Could you check a few things on this model? Use its own coordinates, in mm. A direction names the side the tool comes from. Round coordinates to 2 decimals unless told otherwise and drop trailing zeros. Loops run counter-clockwise (first coordinate to the right, second up) from the corner with the lowest first, then second, coordinate; pieces in that order, holes last.
from build123d import *

# Parameters (mm, degrees)
SKETCH_1_R      = 1.5
EXTRUDE_1_DEPTH = 2.2
FILLET_1_R      = 1


with BuildPart() as part:
    # 草图1 → 凸台-拉伸1 (new body)
    with BuildSketch(Plane(origin=(0, 0, 0), x_dir=(0, 0, -1), z_dir=(1, 0, 0))):
        Polygon((-14.5, -10), (23.5, -10), (23.5, 10), (-14.5, 10), (-14.5, 12), (-21.5, 12), (-21.5, 10), (-23.5, 10), (-23.5, -10), (-21.5, -10), (-21.5, -12), (-14.5, -12), align=None)
        with BuildLine():
            ThreePointArc((-15.845, -6.995), (-16.139357685, -7.705642315), (-16.85, -8))
            Line((-16.85, -8), (-19.15, -8))
            ThreePointArc((-19.15, -8), (-20.155, -6.995), (-19.15, -5.99))
            Line((-19.15, -5.99), (-19.15, 5.99))
            ThreePointArc((-19.15, 5.99), (-20.155, 6.995), (-19.15, 8))
            Line((-19.15, 8), (-16.85, 8))
            ThreePointArc((-16.85, 8), (-16.139357685, 7.705642315), (-15.845, 6.995))
            ThreePointArc((-15.845, 6.995), (-16.139357685, 6.284357685), (-16.85, 5.99))
            Line((-16.85, 5.99), (-16.85, -5.99))
            ThreePointArc((-16.85, -5.99), (-16.139357685, -6.284357685), (-15.845, -6.995))
        make_face(mode=Mode.SUBTRACT)
        with BuildLine():
            Line((10, -7), (-10.85, -7))
            ThreePointArc((-10.85, -7), (-12.275, -5.575), (-10.85, -4.15))
            Line((-10.85, -4.15), (10, -4.15))
            ThreePointArc((10, -4.15), (11.425, -5.575), (10, -7))
        make_face(mode=Mode.SUBTRACT)
        with BuildLine():
            Line((-3.01, -1.15), (-8.99, -1.15))
            ThreePointArc((-8.99, -1.15), (-9.995, -2.155), (-11, -1.15))
            Line((-11, -1.15), (-11, 1.15))
            ThreePointArc((-11, 1.15), (-9.995, 2.155), (-8.99, 1.15))
            Line((-8.99, 1.15), (-3.01, 1.15))
            ThreePointArc((-3.01, 1.15), (-2.005, 2.155), (-1, 1.15))
            Line((-1, 1.15), (-1, -1.15))
            ThreePointArc((-1, -1.15), (-2.005, -2.155), (-3.01, -1.15))
        make_face(mode=Mode.SUBTRACT)
        with Locations((16, -5)):
            Circle(SKETCH_1_R, mode=Mode.SUBTRACT)
        with BuildLine():
            ThreePointArc((-10.85, 4.15), (-12.275, 5.575), (-10.85, 7))
            Line((-10.85, 7), (10, 7))
            ThreePointArc((10, 7), (11.425, 5.575), (10, 4.15))
            Line((10, 4.15), (-10.85, 4.15))
        make_face(mode=Mode.SUBTRACT)
        with BuildLine():
            Line((16.99, -1.15), (11.01, -1.15))
            ThreePointArc((11.01, -1.15), (10.005, -2.155), (9, -1.15))
            Line((9, -1.15), (9, 1.15))
            ThreePointArc((9, 1.15), (10.005, 2.155), (11.01, 1.15))
            Line((11.01, 1.15), (16.99, 1.15))
            ThreePointArc((16.99, 1.15), (17.995, 2.155), (19, 1.15))
            Line((19, 1.15), (19, -1.15))
            ThreePointArc((19, -1.15), (17.995, -2.155), (16.99, -1.15))
        make_face(mode=Mode.SUBTRACT)
        with Locations((16, 5)):
            Circle(SKETCH_1_R, mode=Mode.SUBTRACT)
    extrude(amount=EXTRUDE_1_DEPTH)

    # 圆角1
    fillet_1_edges = [part.edges().sort_by_distance(p)[0] for p in [
        (1.1, -10, 23.5),
        (1.1, 10, 23.5),
        (1.1, 12, 14.5),
        (1.1, 10, 14.5),
        (1.1, 10, -23.5),
        (1.1, -10, -23.5),
        (1.1, -10, 14.5),
        (1.1, -12, 14.5),
        (1.1, -12, 21.5),
        (1.1, -10, 21.5),
        (1.1, 12, 21.5),
        (1.1, 10, 21.5),
    ]]
    fillet(fillet_1_edges, radius=FILLET_1_R - 0.0001)  # a hair under: the kernel refuses the full size


solid = part.part
Item 1: Will these pins go through, and if not, where does the flat tip stop? pin 1 (1.1 mm diameter, centred on x = 1.5, z = 5.5, fed in from -Y); pin 2 (3 mm diameter, centred on y = 3, z = 15.5, fed in from -X); pin 3 (0.7 mm diameter, centred on x = 0.5, z = 5, fed in from +Y).
Results list:
pin 1: stops at y = -10
pin 2: stops at x = 0
pin 3: stops at y = 10
Item 2: If we section it at A-A, the plane z = -8: Please give me the cut outline in (x, y), then the cut area to 3 significant figures.
Results list:
outline: (0, -10) - (2.2, -10) - (2.2, -7) - (0, -7) - close; (0, -4.15) - (2.2, -4.15) - (2.2, 4.15) - (0, 4.15) - close; (0, 7) - (2.2, 7) - (2.2, 10) - (0, 10) - close
area: 31.5 mm2
Item 3: If we section it at D-D, the plane y = -7.5: Please give me the cut outline in (x, z), then the cut area to 3 significant figures.
Results list:
outline: (0, -23.5) - (2.2, -23.5) - (2.2, 15.98) - (0, 15.98) - close; (0, 20.02) - (2.2, 20.02) - (2.2, 23.5) - (0, 23.5) - close
area: 94.5 mm2
Item 4: If we section it at B-B, the plane y = 5: Please give me the cut outline in (x, z), then the cut area to 3 significant figures.
Results list:
outline: (0, -23.5) - (2.2, -23.5) - (2.2, -17.5) - (0, -17.5) - close; (0, -14.5) - (2.2, -14.5) - (2.2, -11.3) - (0, -11.3) - close; (0, 12.15) - (2.2, 12.15) - (2.2, 16.85) - (0, 16.85) - close; (0, 19.15) - (2.2, 19.15) - (2.2, 23.5) - (0, 23.5) - close
area: 40.1 mm2
Item 5: We'd pull the mould along Y, two halves only. Please class faces 3 (the flat face through (1, 0, 19.15)), 4 (the cylindrical face through (1.115, -11.715, 21.199)), 5 (the flat face through (1, 10, -5)): released by +Y, released by -Y, zero draft, split by the parting line, or undercut.
Results list:
face 3: undercut
face 4: released by -Y
face 5: released by +Y
Item 6: If we section it at C-C, the plane z = -16: Please give me the cut outline in (x, y).
Results list:
outline: (0, -10) - (2.2, -10) - (2.2, -6.5) - (0, -6.5) - close; (0, -3.5) - (2.2, -3.5) - (2.2, -1.15) - (0, -1.15) - close; (0, 1.15) - (2.2, 1.15) - (2.2, 3.5) - (0, 3.5) - close; (0, 6.5) - (2.2, 6.5) - (2.2, 10) - (0, 10) - close
Item 7: For faces 1 (the flat face through (1, -12, 18)), 2 (the cylindrical face through (1.085, 6.973, 20.155)), which set-ups out of +Z, -Z, +X, -X, +Y, -Y let a thin tool reach every point of the face, with its end or its side?
Results list:
face 1: +Z, -Z, +X, -X, -Y
face 2: +X, -X
Item 8: If I drill on line 1 along Z through (x, y) = (1.25, 0.25); line 2 along Y through (x, z) = (0.95, -7); line 3 along Y through (x, z) = (2.05, 8.5), over which ranges is the centre line in solid material (lowest first)?
Results list:
line 1: z = -23.5 to -19, -9 to 1, 11 to 16.85, 19.15 to 23.5
line 2: y = -10 to -7, -4.15 to 4.15, 7 to 10
line 3: y = -10 to -7, -4.15 to -1.15, 1.15 to 4.15, 7 to 10
